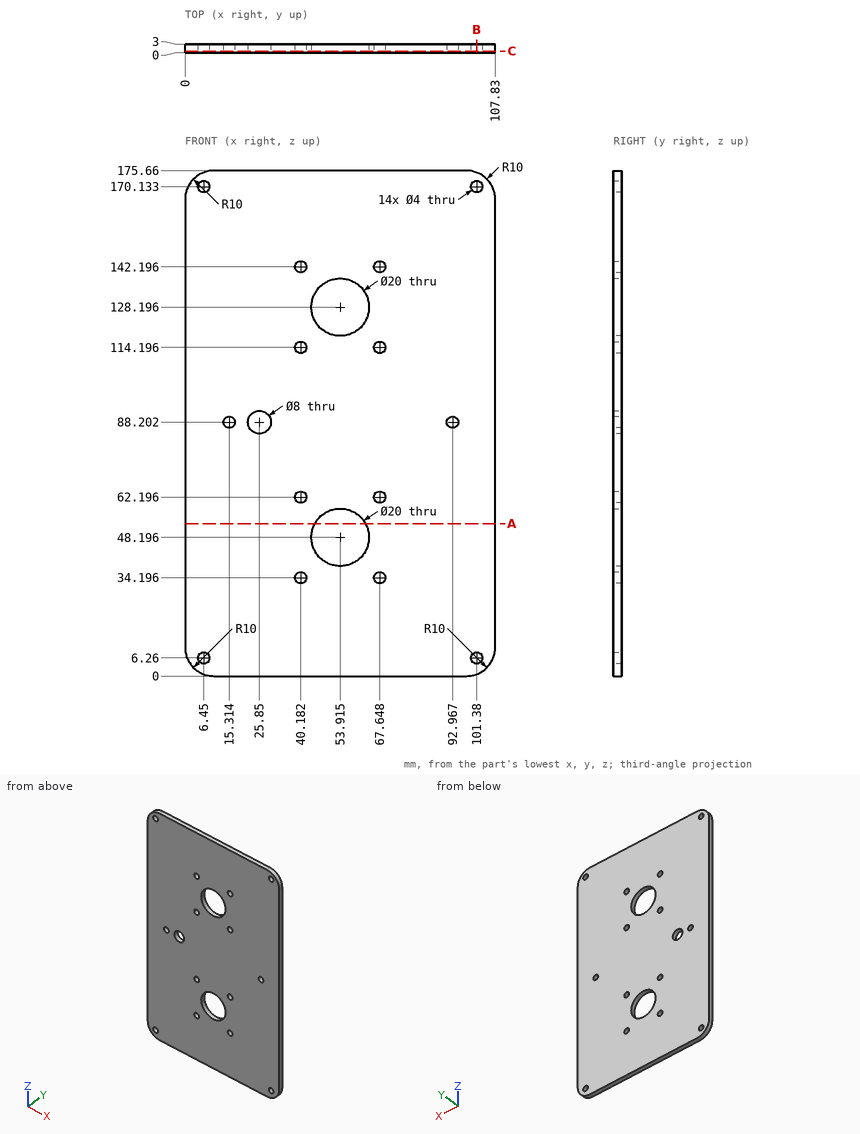
Study the drawing (mm; zero at the part's minimum x, y, z) and answer. Give positions to 0.01 mm unless a question says otherwise; leave off trailing zeros. Loops run counter-clockwise (first coordinate to the right, second up) from the corner with the lowest first, then second, coordinate; pieces in that order, holes last. Notation, with made-up numbers: (60.25, 71) - (70.25, 71) arc R21 ccw to (70.25, 81) - close; hole circle Ø1 at (-6.75, 73). An arc over 180 degrees is marked (long way). Answer as CSV lines item,"result". Start each with the question number.
1) Find section A-A (z = 53). Write down the section's boundary in (x, y) (1 decimal), then the cut area to 3 significant figures.
2) Find section B-B (x = 101.38). Write down the section's boundary in (y, z), then the cut area to 3 significant figures.
3) Find section C-C (y = 0.55). State how many separate pieces and enclosed holes the cut face has, then the cut area to 3 significant figures.
4) Straight lines are drawn through the part: L1, parallel to Z at x = 46, y = 1.9 (1 decimal); L2, parallel to X at y = 0.7, z = 48; L3, parallel to Z at x = 5, y = 1.85 (1 decimal). For each, find the intervals that lie inside material, in ascending order. Write a range as from..to.
Findings below:
1,outline,"(0, 0) - (45.1, 0) - (45.1, 3) - (0, 3) - close; (62.7, 0) - (107.8, 0) - (107.8, 3) - (62.7, 3) - close"
1,area,"271 mm^2"
2,outline,"(0, 0.65) - (3, 0.65) - (3, 4.26) - (0, 4.26) - close; (0, 8.26) - (3, 8.26) - (3, 168.13) - (0, 168.13) - close; (0, 172.13) - (3, 172.13) - (3, 175.01) - (0, 175.01) - close"
2,area,"499 mm^2"
3,separate pieces,"1"
3,enclosed holes,"17"
3,area,"18,000 mm^2"
4,L1,"0..42.1, 54.3..122.1, 134.3..175.7"
4,L2,"0..43.92, 63.91..107.83"
4,L3,"1.3..4.9, 7.6..168.8, 171.5..174.3"
